Autodesk Inventor part; units mm, degrees
ref_plane "YZ Plane" through (0, 0, 0) normal (1, 0, 0) x (0, 1, 0)
ref_plane "XZ Plane" through (0, 0, 0) normal (0, 1, 0) x (-1, 0, 0)
ref_plane "XY Plane" through (0, 0, 0) normal (0, 0, 1) x (1, 0, 0)
sketch "Sketch1" plane through (0, 0, 0) normal (0, 0, 1) x (1, 0, 0)
  line L0 (-22.5, 0) -> (22.5, 0)
  line L1 (22.5, 0) -> (22.5, 25)
  line L2 (22.5, 25) -> (12.5, 25)
  line L3 (12.5, 25) -> (12.5, 15)
  line L4 (12.5, 15) -> (-12.5, 15)
  line L5 (-12.5, 15) -> (-12.5, 25)
  line L6 (-12.5, 25) -> (-22.5, 25)
  line L7 (-22.5, 25) -> (-22.5, 0)
  point P0 (0, 0)
  point P1 (0, 0)
  dimension "d0" = 45
  dimension "d1" = 25
  dimension "d2" = 10
  dimension "d3" = 10
extrude "Extrusion1" add sketch "Sketch1" along normal mid plane 15
sketch "Sketch3" plane through (0, 0, 7.5) normal (0, 0, 1) x (1, 0, 0)
  line L0 (12.5, 7) -> (-12.5, 7) construction
  line L1 (0, 0) -> (0, 14) construction
  line L2 (12.5, 15) -> (-12.5, 15)
  point P0 (0, 7)
  dimension "d14" = 8
  dimension "d15" = 25
hole "Hole2" at (12.5, 7, 7.5) at (-12.5, 7, 7.5) direction (0, 0, -1) diameter 4 end through all
properties part number "sujetador inferior"
Work out the finished part from the listing and answer in its coordinate system (mm). A direction names the side the tool comes from. Coordinates: 2 decimals unless noted, no trailing zeros. Order: outer loops, then holes, each group sorted by start corner. A loop starts at its lowest first (then second) coordinate and runs counter-clockwise, first axis right, second up. Notation, with made-up numbers: (84.5, 59.25) - (91.5, 59.25) arc R11 cw to (91.5, 68.25) - close; hole circle Ø4 at (88.25, 76). An arc over 180 degrees is marked (long way). Put each result on its own line as item: value. Start each with the question number.
1) A flat-ended cylindrical pin translates along its axis: pin 1 (1.5 mm diameter, centred on x = -6.5, z = 3, fed in from +Y). Find the tip coordinate at first contact, or state that the pin passes through.
2) Find section B-B (y = 7). Give the vertices of the cut face in (x, z), plus the area to 3 significant figures.
3) For faces 1 (the flat face through (-12.5, 20, 0)), 2 (the cylindrical face through (11.148, 8.474, -0.105)), determine the directions among +Z, -Z, +X, -X, +Y, -Y from which every point of the face is accessible in a straight line to the end or side of a thin tool.
4) Find the intervals of material crossed by line 1 (X direction, y = 7, z = 0.5); line 2 (X direction, y = 20.25, z = 6.5); line 3 (X direction, y = 8.5, z = 5.5), in increasing order. Write a range as from..to.
5) Find section C-C (x = 0). Give the vertices of the cut face in (y, z).
6) For a pull along X with two mould halves and no side action, classify faces 3 (the flat face through (0, 15, 0)), 4 (the flat face through (-17, 25, 0)), 5 (the flat face through (22.5, 12, 0)) as released by +X, released by -X, zero draft, split by the parting line, or undercut.
7) Find section A-A (z = -5). Give the vertices of the cut face in (x, y).
Results list:
1. pin 1: stops at y = 15
2. outline: (-22.5, -7.5) - (-14.5, -7.5) - (-14.5, 7.5) - (-22.5, 7.5) - close; (-10.5, -7.5) - (10.5, -7.5) - (10.5, 7.5) - (-10.5, 7.5) - close; (14.5, -7.5) - (22.5, -7.5) - (22.5, 7.5) - (14.5, 7.5) - close
2. area: 555 mm^2
3. face 1: +Z, -Z, +Y
3. face 2: +Z, -Z
4. line 1: x = -22.5..-14.5, -10.5..10.5, 14.5..22.5
4. line 2: x = -22.5..-12.5, 12.5..22.5
4. line 3: x = -22.5..-13.82, -11.18..11.18, 13.82..22.5
5. outline: (0, -7.5) - (15, -7.5) - (15, 7.5) - (0, 7.5) - close
6. face 3: undercut
6. face 4: zero draft
6. face 5: released by +X
7. outline: (-22.5, 0) - (22.5, 0) - (22.5, 25) - (12.5, 25) - (12.5, 15) - (-12.5, 15) - (-12.5, 25) - (-22.5, 25) - close; hole circle Ø4 at (-12.5, 7); hole circle Ø4 at (12.5, 7)
